from build123d import *

# Parameters (mm, degrees)
SKETCH1_R               = 3
BOSS_EXTRUDE1_DEPTH     = 275
SKETCH3_W               = 0.8
SKETCH3_H               = 0.5
CUT_EXTRUDE2_DEPTH      = 276.032725326
CUT_EXTRUDE2_DEPTH_BACK = 276.032725326
SKETCH4_W               = 3.470061058
SKETCH4_H               = 7
SKETCH4_W_2             = 2.92528695
CHAMFER1_SIZE           = 0.3


with BuildPart() as part:
    # Sketch1 → Boss-Extrude1 (new body)
    with BuildSketch(Plane.XY):
        Circle(SKETCH1_R)
    extrude(amount=BOSS_EXTRUDE1_DEPTH)

    # Sketch3 → Cut-Revolve1 (revolve, cut)
    with BuildSketch(Plane(origin=(0, 0, 0), x_dir=(0, 0, -1), z_dir=(1, 0, 0)), mode=Mode.PRIVATE) as cut_revolve1_sk:
        with Locations((-266.6, 2.75)):
            Rectangle(SKETCH3_W, SKETCH3_H)
        with Locations((-260.65, 2.75)):
            Rectangle(SKETCH3_W, SKETCH3_H)
        with Locations((-13.4, 2.75)):
            Rectangle(SKETCH3_W, SKETCH3_H)
        with Locations((-7.45, 2.75)):
            Rectangle(SKETCH3_W, SKETCH3_H)
    revolve(cut_revolve1_sk.sketch.rotate(Axis((0, 0, 263.365004794), (0, 0, -1)), 90), axis=Axis((0, 0, 263.365004794), (0, 0, -1)), mode=Mode.SUBTRACT)

    # Sketch4 → Cut-Extrude2 (cut, two sides: drawn at the far end of the back side and taken through both)
    with BuildSketch(Plane(origin=(0, 0, 0), x_dir=(1, 0, 0), z_dir=(0, 1, 0)).offset(-CUT_EXTRUDE2_DEPTH_BACK)):
        with Locations((4.235030529, -3.5)):
            Rectangle(SKETCH4_W, SKETCH4_H)
        with Locations((-3.962643475, -3.5)):
            Rectangle(SKETCH4_W_2, SKETCH4_H)
    extrude(amount=CUT_EXTRUDE2_DEPTH + CUT_EXTRUDE2_DEPTH_BACK, mode=Mode.SUBTRACT)

    # Chamfer1
    chamfer1_edges = [part.edges().sort_by_distance(p)[0] for p in [
        (0, 3, 0),
        (0, -3, 0),
    ]]
    chamfer(chamfer1_edges, length=CHAMFER1_SIZE)


solid = part.part
Build history of the part. All positions in model axes, mm. A direction names the side the tool comes from. Round coordinates to 2 decimals unless told otherwise and drop trailing zeros. Write each loop counter-clockwise with the first axis right and the second up, starting at its lowest first coordinate (ties: lowest second). Pieces come first, ordered by that corner, then holes. Notation, with made-up numbers: M -15.75,54.25 L 38.25,54.25 A29 ccw 38.25,76.25 Z; hole C 49,68 d6. An arc over 180 degrees is marked long. Answer in a Markdown table with one row per item.
1. Probe L1, parallel to Z at x = -2.25, y = 1.35; L2, parallel to Y at x = -1.65, z = 255; L3, parallel to Y at x = -0.3, z = 149. List the from-to ranges inside material, lowest first. Write a range as [from, to].
Geometry check:
| item | result |
|---|---|
| L1 | [0, 7.05], [7.85, 13], [13.8, 260.25], [261.05, 266.2], [267, 275] |
| L2 | [-2.51, 2.51] |
| L3 | [-2.98, 2.98] |
2. Flat gauge pins, fed straight in: P1, Ø1.7, axis at y = -1, z = 4, coming from the -X side; P2, Ø1.7, axis at y = -0.5, z = 4, coming from the +X side; P3, Ø2, axis at y = 1.5, z = 116, coming from the -X side. Where does each tip first touch, or does it go through?
Geometry check:
| item | result |
|---|---|
| P1 | x = -2.5 |
| P2 | x = 2.5 |
| P3 | x = -2.96 |
3. Which spindle directions (+Z, -Z, +X, -X, +Y, -Y) get a long thin tool onto all of the face, cutting with end or side? Do faces 1 (the face through (-2.5, -0.1, 13.4)), 2 (the face through (-3, 0, 264)). Say none if no direction does.
Geometry check:
| item | result |
|---|---|
| face 1 | none |
| face 2 | +Z, -Z |
4. Saw through at A-A (z = 189). List the corners of the cut face in (x, y), and give its area (3 significant figures).
Geometry check:
| item | result |
|---|---|
| outline | C 0,0 d6 |
| area | 28.3 mm2 |
5. Mould opens along Z. For faces 3 (the face through (0, 0, 0)), 4 (the face through (2, -2, 261.05)), 5 (the face through (-3, 0, 271)) say: +Z half, -Z half, draft (parallel to the pull), parting line (faces both ways), or undercut.
Geometry check:
| item | result |
|---|---|
| face 3 | -Z half |
| face 4 | undercut |
| face 5 | draft |
